Design review of the part built by this model. Coordinates are the model's own, in mm. A direction names the side the tool comes from. Coordinates: 2 decimals unless noted, no trailing zeros. Loops run counter-clockwise (first coordinate to the right, second up) from the corner with the lowest first, then second, coordinate; pieces in that order, holes last. Notation, with made-up numbers: (-8, 51.25) - (37, 51.25) arc R25 cw to (37, 65.25) - close; hole circle Ø5 at (-12.5, 57.5). An arc over 180 degrees is marked (long way). Return JSON: item names as keys, results as strings. Group by question number.
from build123d import *

# Parameters (mm, degrees)
RESSALTO_EXTRUS_O1_DEPTH = 5.5
ESBO_O2_R                = 19
CORTE_EXTRUS_O1_DEPTH    = 8.55
CORTE_EXTRUS_O2_DEPTH    = 3.45
ESBO_O4_R                = 1.6
CORTE_EXTRUS_O3_DEPTH    = 12
ESBO_O5_R                = 2.8
CORTE_EXTRUS_O4_DEPTH    = 3


with BuildPart() as part:
    # Esboço1 → Ressalto-extrusão1 (new body, symmetric)
    with BuildSketch(Plane(origin=(0, 0, 0), x_dir=(1, 0, 0), z_dir=(0, 1, 0))):
        with BuildLine():
            Line((-16.1, -20.1), (16.1, -20.1))
            ThreePointArc((16.1, -20.1), (18.928427125, -18.928427125), (20.1, -16.1))
            Line((20.1, -16.1), (20.1, 16.1))
            ThreePointArc((20.1, 16.1), (18.928427125, 18.928427125), (16.1, 20.1))
            Line((16.1, 20.1), (-16.1, 20.1))
            ThreePointArc((-16.1, 20.1), (-18.928427125, 18.928427125), (-20.1, 16.1))
            Line((-20.1, 16.1), (-20.1, -16.1))
            ThreePointArc((-20.1, -16.1), (-18.928427125, -18.928427125), (-16.1, -20.1))
        make_face()
    extrude(amount=RESSALTO_EXTRUS_O1_DEPTH, both=True)

    # Esboço2 → Corte-extrusão1 (cut)
    with BuildSketch(Plane(origin=(0, 5.5, 0), x_dir=(1, 0, 0), z_dir=(0, 1, 0))):
        Circle(ESBO_O2_R)
    extrude(amount=-CORTE_EXTRUS_O1_DEPTH, mode=Mode.SUBTRACT)

    # Esboço3 → Corte-extrusão2 (cut, through all)
    with BuildSketch(Plane(origin=(0, -3.05, 0), x_dir=(1, 0, 0), z_dir=(0, 1, 0))):
        with BuildLine():
            Line((1.5, 10.897247359), (1.5, 18.940696925))
            ThreePointArc((1.5, 18.940696925), (16.454482672, 9.5), (17.153124702, -8.171310357))
            Line((17.153124702, -8.171310357), (10.187293044, -4.149585574))
            ThreePointArc((10.187293044, -4.149585574), (9.526279442, 5.5), (1.5, 10.897247359))
        make_face()
        with BuildLine():
            Line((-1.5, 10.897247359), (-1.5, 18.940696925))
            ThreePointArc((-1.5, 18.940696925), (-16.454482672, 9.5), (-17.153124702, -8.171310357))
            Line((-17.153124702, -8.171310357), (-10.187293044, -4.149585574))
            ThreePointArc((-10.187293044, -4.149585574), (-9.526279442, 5.5), (-1.5, 10.897247359))
        make_face()
        with BuildLine():
            Line((8.687293044, -6.747661785), (15.653124702, -10.769386568))
            ThreePointArc((15.653124702, -10.769386568), (0, -19), (-15.653124702, -10.769386568))
            Line((-15.653124702, -10.769386568), (-8.687293044, -6.747661785))
            ThreePointArc((-8.687293044, -6.747661785), (0, -11), (8.687293044, -6.747661785))
        make_face()
    extrude(amount=-CORTE_EXTRUS_O2_DEPTH, mode=Mode.SUBTRACT)

    # Esboço4 → Corte-extrusão3 (cut, through all)
    with BuildSketch(Plane.XZ.offset(5.5)):
        with Locations((-16.1, 16.1)):
            Circle(ESBO_O4_R)
        with Locations((16.1, 16.1)):
            Circle(ESBO_O4_R)
        with Locations((16.1, -16.1)):
            Circle(ESBO_O4_R)
        with Locations((-16.1, -16.1)):
            Circle(ESBO_O4_R)
    extrude(amount=-CORTE_EXTRUS_O3_DEPTH, mode=Mode.SUBTRACT)

    # Esboço5 → Corte-extrusão4 (cut)
    with BuildSketch(Plane(origin=(0, 5.5, 0), x_dir=(1, 0, 0), z_dir=(0, 1, 0))):
        with Locations((-16.1, 16.1)):
            Circle(ESBO_O5_R)
        with Locations((-16.1, -16.1)):
            Circle(ESBO_O5_R)
        with Locations((16.1, -16.1)):
            Circle(ESBO_O5_R)
        with Locations((16.1, 16.1)):
            Circle(ESBO_O5_R)
    extrude(amount=-CORTE_EXTRUS_O4_DEPTH, mode=Mode.SUBTRACT)


solid = part.part
Item 1: For faces 4 (the face through (13.72, -4.26, 6.19)), 5 (the face through (18.959, 0.077, -18.897)), 6 (the face through (16, 2.5, -14)), list the 3-axis set-ups (+Z, -Z, +X, -X, +Y, -Y) from which the entire face can be reached by the end or side of a thin tool; tool diameter is ignored.
Item 2: Add section A-A (z = 0). State the section outline as (x, y) points.
Item 3: Add section B-B (x = 0). State the section outline as (y, z) points.
Item 4: For P1, Ø1.5, axis at x = -12.5, z = -11, coming from the +Y side; P2, Ø2, axis at x = -1, z = 7.5, coming from the +Y side; P3, Ø4.5, axis at x = 16.5, z = 16, coming from the +Y side, all flat-tipped, find the tip position at first contact; note any pin that passes through.
Item 5: Add section D-D (x = -12). State the section outline as (y, z) points.
Item 6: To check wall thickness, follow line 1 (X direction, y = 3.6, z = -16.1); line 2 (Z direction, x = 17, y = -0.25); line 3 (Z direction, x = 16, y = -1). State the ranges of each line that lie inside material, in increasing order. Write a range as from..to.
Item 7: Add section C-C (y = 4). State the section outline as (x, z) points, then the cut area to 3 significant figures.
Item 8: Draft analysis for pull direction X (two halves, no side actions). For faces 1 (the face through (-12, 5.5, -15)), 2 (the face through (15.75, -1.56, -17.66)), 3 (the face through (-20.1, 0, 0)), state which applies: pulls with the +X half, pulls with the -X half, needs draft (parallel to the pull), parting line crosses it, or undercut.
Answers below:
{
 "1": {"face 4": "+Y, -Y", "face 5": "-Z, +X, +Y, -Y", "face 6": "+Y"},
 "2": {"outline": "(-20.1, -5.5) - (-19, -5.5) - (-19, 5.5) - (-20.1, 5.5) - close; (-11, -5.5) - (11, -5.5) - (11, -3.05) - (-11, -3.05) - close; (19, -5.5) - (20.1, -5.5) - (20.1, 5.5) - (19, 5.5) - close"},
 "3": {"outline": "(-5.5, -20.1) - (5.5, -20.1) - (5.5, -19) - (-3.05, -19) - (-3.05, 11) - (-5.5, 11) - close; (-5.5, 19) - (5.5, 19) - (5.5, 20.1) - (-5.5, 20.1) - close"},
 "4": {"P1": "passes through", "P2": "stops at y = -3.05", "P3": "stops at y = 2.5"},
 "5": {"outline": "(-5.5, -20.1) - (5.5, -20.1) - (5.5, -14.73) - (-5.5, -14.73) - close; (-5.5, 5.2) - (-3.05, 5.2) - (-3.05, 8.66) - (-5.5, 8.66) - close; (-5.5, 14.73) - (5.5, 14.73) - (5.5, 20.1) - (-5.5, 20.1) - close"},
 "6": {"line 1": "x = -20.1..-18.9, -13.3..-10.09, 10.09..13.3, 18.9..20.1", "line 2": "z = -20..-17.42, -14.78..-8.49, 8.49..14.78, 17.42..20", "line 3": "z = -20.1..-17.7, -14.5..-10.25, 10.25..14.5, 17.7..20.1"},
 "7": {"outline": "(-20.1, -16.1) arc R4 ccw to (-16.1, -20.1) - (16.1, -20.1) arc R4 ccw to (20.1, -16.1) - (20.1, 16.1) arc R4 ccw to (16.1, 20.1) - (-16.1, 20.1) arc R4 ccw to (-20.1, 16.1) - close; hole circle Ø38 at (0, 0); hole circle Ø5.6 at (-16.1, -16.1); hole circle Ø5.6 at (-16.1, 16.1); hole circle Ø5.6 at (16.1, -16.1); hole circle Ø5.6 at (16.1, 16.1)", "area": "370 mm^2"},
 "8": {"face 1": "needs draft", "face 2": "undercut", "face 3": "pulls with the -X half"}
}
